from build123d import *

# Parameters (mm, degrees)
BOSS_EXTRUDE1_DEPTH      = 6.75
BOSS_EXTRUDE1_DEPTH_BACK = 6.75
SKETCH1_W                = 13.2
SKETCH1_H                = 13.5
SKETCH2_W                = 3.16
SKETCH2_H                = 23
SKETCH3_W                = 3.16
SKETCH3_H                = 23
SKETCH4_W                = 15
SKETCH4_H                = 3.61


with BuildPart() as part:
    # Sketch1 → Boss-Extrude1 (new, two sides: drawn at the far end of the back side and taken through both)
    with BuildSketch(Plane.XY.offset(-BOSS_EXTRUDE1_DEPTH_BACK)):
        with Locations((26, 0)):
            Rectangle(SKETCH1_W, SKETCH1_H)
    extrude(amount=BOSS_EXTRUDE1_DEPTH + BOSS_EXTRUDE1_DEPTH_BACK)

    # Sketch2 → Revolve1 (revolve)
    with BuildSketch(Plane.XY, mode=Mode.PRIVATE) as revolve1_sk:
        with Locations((27.58, 0)):
            Rectangle(SKETCH2_W, SKETCH2_H)
    revolve(revolve1_sk.sketch.rotate(Axis((26, -11.5, 0), (0, 1, 0)), 270), axis=Axis((26, -11.5, 0), (0, 1, 0)))

    # Sketch3 → Revolve2 (revolve)
    with BuildSketch(Plane(origin=(0, 0, 0), x_dir=(1, 0, 0), z_dir=(0, 1, 0)), mode=Mode.PRIVATE) as revolve2_sk:
        with Locations((27.58, 0)):
            Rectangle(SKETCH3_W, SKETCH3_H)
    revolve(revolve2_sk.sketch.rotate(Axis((26, 0, 11.5), (0, 0, -1)), 180), axis=Axis((26, 0, 11.5), (0, 0, -1)))

    # Sketch4 → Revolve3 (revolve)
    with BuildSketch(Plane.XY, mode=Mode.PRIVATE) as revolve3_sk:
        with Locations((26, 1.805)):
            Rectangle(SKETCH4_W, SKETCH4_H)
    revolve(revolve3_sk.sketch.rotate(Axis((33.5, 0, 0), (-1, 0, 0)), 270), axis=Axis((33.5, 0, 0), (-1, 0, 0)))


solid = part.part
Read the model definition and answer for the solid it produces. Units are mm, in the model's axes. A direction names the side the tool comes from. Coordinates: 2 decimals unless noted, no trailing zeros. Loops run counter-clockwise (first coordinate to the right, second up) from the corner with the lowest first, then second, coordinate; pieces in that order, holes last.
Q1. The part is cut by section D-D on y = 4. Write down the section's boundary in (x, z).
Q2. Which of the six approach directions +Z, -Z, +X, -X, +Y, -Y give full straight-line access (tool end or side, diameter ignored) to faces 1 (the face through (18.956, -1.383, 3.335)), 2 (the face through (29, 2, -6.75)), 3 (the face through (23.197, 9.158, 1.458)), 4 (the face through (29, -6.75, -2)), 5 (the face through (29, 2, 6.75))?
Q3. Consider probe 1 along Y at (x, z) = (22.25, -2); probe 2 along X at (y, z) = (-3, -4.5). Determine where each line is inside the solid, lowest interval first.
Q4. The part is cut by section A-A on z = 0. Write down the section's boundary in (x, y), and give its area (3 significant figures).
Q5. Each of these flat-tipped pins is pushed along its axis until it touches: pin 1 Ø2 at (x, y) = (25, 7) entering from -Z; pin 2 Ø1 at (x, y) = (23.5, -8.5) entering from -Z; pin 3 Ø1 at (y, z) = (-7, -5) entering from -X. Where does it stop, or does it pass through?
Q6. The part is cut by section C-C on x = 21.25. Write down the section's boundary in (y, z), and give its area (3 significant figures).
Results below:
1. outline: (19.4, -6.75) - (32.6, -6.75) - (32.6, 6.75) - (19.4, 6.75) - close
2. face 1: -X
2. face 2: -Z
2. face 3: +Y
2. face 4: -Y
2. face 5: +Z
3. probe 1: y = -6.75 to 6.75
3. probe 2: x = 19.4 to 32.6
4. outline: (18.5, -3.61) - (19.4, -3.61) - (19.4, -6.75) - (22.84, -6.75) - (22.84, -11.5) - (29.16, -11.5) - (29.16, -6.75) - (32.6, -6.75) - (32.6, -3.61) - (33.5, -3.61) - (33.5, 3.61) - (32.6, 3.61) - (32.6, 6.75) - (29.16, 6.75) - (29.16, 11.5) - (22.84, 11.5) - (22.84, 6.75) - (19.4, 6.75) - (19.4, 3.61) - (18.5, 3.61) - close
4. area: 251 mm2
5. pin 1: stops at z = -6.75
5. pin 2: stops at z = -2.45
5. pin 3: stops at x = 19.4
6. outline: (-6.75, -6.75) - (6.75, -6.75) - (6.75, 6.75) - (-6.75, 6.75) - close
6. area: 182 mm2
